from build123d import *

# Parameters (mm, degrees)
BOSS_EXTRUDE1_START = 650
SKETCH1_W           = 1906
SKETCH1_H           = 1006
BOSS_EXTRUDE1_DEPTH = 2
SKETCH2_W           = 1906
SKETCH2_H           = 1006
SKETCH2_W_2         = 1900
SKETCH2_H_2         = 1002.833158448
BOSS_EXTRUDE2_DEPTH = 648
FILLET1_R           = 100
SKETCH3_W           = 1400
SKETCH3_H           = 560
CUT_EXTRUDE1_DEPTH  = 143


with BuildPart() as part:
    # Sketch1 → Boss-Extrude1 (new body)
    with BuildSketch(Plane(origin=(0, 0, 0), x_dir=(1, 0, 0), z_dir=(0, 1, 0)).offset(BOSS_EXTRUDE1_START)):
        Rectangle(SKETCH1_W, SKETCH1_H)
    extrude(amount=BOSS_EXTRUDE1_DEPTH)

    # Sketch2 → Boss-Extrude2 (add)
    with BuildSketch(Plane.XZ.offset(-650)):
        Rectangle(SKETCH2_W, SKETCH2_H)
        Rectangle(SKETCH2_W_2, SKETCH2_H_2, mode=Mode.SUBTRACT)
    extrude(amount=BOSS_EXTRUDE2_DEPTH)

    # Fillet1
    fillet1_edges = [part.edges().sort_by_distance(p)[0] for p in [
        (953, 652, 0),
        (0, 652, -503),
        (0, 650, 501.416579224),
        (-950, 650, 0),
        (0, 650, -501.416579224),
        (950, 650, 0),
        (-953, 652, 0),
        (0, 652, 503),
    ]]
    fillet(fillet1_edges, radius=FILLET1_R)

    # Sketch3 → Cut-Extrude1 (cut)
    with BuildSketch(Plane(origin=(0, 0, -503), x_dir=(-1, 0, 0), z_dir=(0, 0, -1))):
        with Locations((0, 2)):
            Rectangle(SKETCH3_W, SKETCH3_H)
    extrude(amount=-CUT_EXTRUDE1_DEPTH, mode=Mode.SUBTRACT)


solid = part.part
Can you work these out from the model? Positions are in its coordinate system, mm. A direction names the side the tool comes from. Give positions to 0.01 mm unless a question says otherwise; leave off trailing zeros. Write each loop counter-clockwise with the first axis right and the second up, starting at its lowest first coordinate (ties: lowest second). Pieces come first, ordered by that corner, then holes. Notation, with made-up numbers: (42, 61.5) -> (51, 61.5) arc R27 cw to (51, 89.5) -> close; hole circle Ø10 at (-34, 11). An arc over 180 degrees is marked (long way). Answer as a JSON object with one key per item and string values. Group by question number.
Item 1: Please list where these lines run through material, in increasing order: line 1 (Z direction, x = -241, y = 494); line 2 (X direction, y = 271.5, z = -133.5); line 3 (Z direction, x = -79.5, y = 243). Write a range as [from, to].
Item 2: I'm going to push flat-ended pins straight in: P1, Ø0.8, axis at x = -174, z = -502.5, coming from the -Y side; P2, Ø12, axis at x = 537, z = 245, coming from the -Y side. Where does each tip first touch, or does it pass through?
Item 3: Suppose I cut it at C-C (x = 746.5). Please give me the cut outline in (y, z), plus the area to 3 significant figures.
Item 4: For faces 4 (the face through (-13, 403, -503)), 5 (the face through (950, 280, -7)), which set-ups out of +Z, -Z, +X, -X, +Y, -Y let a thin tool reach every point of the face, with its end or its side?
Item 5: We'd pull the mould along Z, two halves only. Please class faces 1 (the face through (-924.484, 621.929, -7.042)), 2 (the face through (13.342, 623.484, 472.929)), 3 (the face through (13.3, 621.48, -471.35)): +Z half, -Z half, draft (parallel to the pull), parting line (faces both ways), or undercut.
Item 6: Suppose I cut it at A-A (z = 342.5). Please give me the cut outline in (x, y).
Item 7: Suppose I cut it at B-B (y = 318). Please give me the cut outline in (x, z), plus the area to 3 significant figures.
Findings:
{
 "1": {"line 1": "z = [-503, -501.42], [501.42, 503]", "line 2": "x = [-953, -950], [950, 953]", "line 3": "z = [501.42, 503]"},
 "2": {"P1": "stops at y = 282", "P2": "stops at y = 650"},
 "3": {"outline": "(2, -503) -> (552, -503) arc R100 ccw to (652, -403) -> (652, 403) arc R100 ccw to (552, 503) -> (2, 503) -> (2, 501.42) -> (550, 501.42) arc R100 cw to (650, 401.42) -> (650, -401.42) arc R100 cw to (550, -501.42) -> (2, -501.42) -> close", "area": "4,060 mm²"},
 "4": {"face 4": "-Z, +X, -X, +Y, -Y", "face 5": "-Y"},
 "5": {"face 1": "draft", "face 2": "+Z half", "face 3": "undercut"},
 "6": {"outline": "(-953, 2) -> (-950, 2) -> (-950, 550) arc R100 cw to (-850, 650) -> (850, 650) arc R100 cw to (950, 550) -> (950, 2) -> (953, 2) -> (953, 552) arc R100 ccw to (853, 652) -> (-853, 652) arc R100 ccw to (-953, 552) -> close"},
 "7": {"outline": "(-953, -503) -> (953, -503) -> (953, 503) -> (-953, 503) -> close; hole (-950, -501.42) -> (950, -501.42) -> (950, 501.42) -> (-950, 501.42) -> close", "area": "12,100 mm²"}
}
